from build123d import *

# Parameters (mm, degrees)
SKETCH1_W           = 100
SKETCH1_H           = 80
BOSS_EXTRUDE1_DEPTH = 30
SKETCH2_W           = 23.5
SKETCH2_H           = 28.5
SKETCH2_W_2         = 27
CUT_EXTRUDE1_DEPTH  = 25
SKETCH3_W           = 80
SKETCH3_H           = 60
CUT_EXTRUDE2_DEPTH  = 3
SKETCH5_W           = 89
SKETCH5_H           = 69
SKETCH5_W_2         = 80
SKETCH5_H_2         = 60
BOSS_EXTRUDE2_DEPTH = 7
FILLET1_R           = 3


with BuildPart() as part:
    # Sketch1 → Boss-Extrude1 (new body)
    with BuildSketch(Plane(origin=(0, 0, 0), x_dir=(1, 0, 0), z_dir=(0, 1, 0))):
        Rectangle(SKETCH1_W, SKETCH1_H)
    extrude(amount=BOSS_EXTRUDE1_DEPTH)

    # Sketch2 → Cut-Extrude1 (cut)
    with BuildSketch(Plane(origin=(0, 30, 0), x_dir=(1, 0, 0), z_dir=(0, 1, 0))):
        with Locations((-28.25, 15.75)):
            Rectangle(SKETCH2_W, SKETCH2_H)
        with Locations((0, 15.75)):
            Rectangle(SKETCH2_W_2, SKETCH2_H)
        with Locations((28.25, 15.75)):
            Rectangle(SKETCH2_W, SKETCH2_H)
        with Locations((28.25, -15.75)):
            Rectangle(SKETCH2_W, SKETCH2_H)
        with Locations((0, -15.75)):
            Rectangle(SKETCH2_W_2, SKETCH2_H)
        with Locations((-28.25, -15.75)):
            Rectangle(SKETCH2_W, SKETCH2_H)
    extrude(amount=-CUT_EXTRUDE1_DEPTH, mode=Mode.SUBTRACT)

    # Sketch3 → Cut-Extrude2 (cut)
    with BuildSketch(Plane(origin=(0, 30, 0), x_dir=(1, 0, 0), z_dir=(0, 1, 0))):
        Rectangle(SKETCH3_W, SKETCH3_H)
    extrude(amount=-CUT_EXTRUDE2_DEPTH, mode=Mode.SUBTRACT)

    # Sketch5 → Boss-Extrude2 (add)
    with BuildSketch(Plane(origin=(0, 30, 0), x_dir=(1, 0, 0), z_dir=(0, 1, 0))):
        Rectangle(SKETCH5_W, SKETCH5_H)
        Rectangle(SKETCH5_W_2, SKETCH5_H_2, mode=Mode.SUBTRACT)
    extrude(amount=BOSS_EXTRUDE2_DEPTH)

    # Fillet1
    fillet1_edges = [part.edges().sort_by_distance(p)[0] for p in [
        (-44.5, 33.5, -34.5),
        (-44.5, 33.5, 34.5),
        (44.5, 33.5, 34.5),
        (44.5, 33.5, -34.5),
    ]]
    fillet(fillet1_edges, radius=FILLET1_R)


solid = part.part
Verification items for the finished model (mm, model axes). A direction names the side the tool comes from. Coordinates: 2 decimals unless noted, no trailing zeros. Order: outer loops, then holes, each group sorted by start corner. A loop starts at its lowest first (then second) coordinate and runs counter-clockwise, first axis right, second up. Notation, with made-up numbers: M 60,39.5 L 84,39.5 A18 ccw 84,62.5 Z; hole C 73,5 d5. An arc over 180 degrees is marked long. One line per item, written item: value. Start each with the question number.
Item 1: Access from +Z, -Z, +X, -X, +Y, -Y to the whole of each face (thin tool, end or side, straight path). Record for faces 4 (the flat face through (-1, 15, 40)), 5 (the flat face through (44.5, 33, 0)), 6 (the flat face through (-44.5, 33, 0)), 7 (the cylindrical face through (-43.64, 33.55, -33.6)), 8 (the flat face through (-13.5, 16, 16)).
Item 2: Sectioned sample at B-B on y = 28.5. Record the cut outline in (x, z), then the cut area to 3 significant figures.
Item 3: Thickness scan on probe 1 along Z at (x, y) = (-17, 8); probe 2 along X at (y, z) = (13.5, -20.5); probe 3 along Z at (x, y) = (13, 28). Record the ranges inside material, lowest first.
Item 4: Mould release check, pull along X, two halves, no side actions. Record for faces 1 (the cylindrical face through (43.64, 33.55, -33.6)), 2 (the flat face through (-1, 33, 34.5)), 3 (the flat face through (0, 27, 0)): pulls with the +X half, pulls with the -X half, needs draft (parallel to the pull), parting line crosses it, or undercut.
Item 5: Sectioned sample at A-A on y = 18.5. Record the cut outline in (x, z), then the cut area to 3 significant figures.
Item 6: Depth check by flat-ended pin: P1, Ø4, axis at x = 15, z = -9.5, coming from the +Y side; P2, Ø12, axis at x = -24.5, z = 14.5, coming from the +Y side; P3, Ø3.5, axis at x = 15, y = 34.5, coming from the +Z side. Enter the tip coordinate at first touch or a pass-through.
Item 7: Sectioned sample at C-C on z = -4.5. Record the cut outline in (x, y), then the cut area to 4 significant figures.
Item 8: Sectioned sample at D-D on x = 4. Record the cut outline in (y, z).
Calculated:
1. face 4: +Z, +X, -X, +Y, -Y
1. face 5: +Z, -Z, +X, +Y
1. face 6: +Z, -Z, -X, +Y
1. face 7: -Z, -X, +Y
1. face 8: +Y
2. outline: M -50,-40 L 50,-40 L 50,40 L -50,40 Z; hole M -40,-30 L 40,-30 L 40,30 L -40,30 Z
2. area: 3,200 mm^2
3. probe 1: -40 to -30, -1.5 to 1.5, 30 to 40
3. probe 2: -50 to -40, -16.5 to -13.5, 13.5 to 16.5, 40 to 50
3. probe 3: -40 to -30, 30 to 40
4. face 1: pulls with the +X half
4. face 2: needs draft
4. face 3: undercut
5. outline: M -50,-40 L 50,-40 L 50,40 L -50,40 Z; hole M -40,-30 L -16.5,-30 L -16.5,-1.5 L -40,-1.5 Z; hole M -40,1.5 L -16.5,1.5 L -16.5,30 L -40,30 Z; hole M -13.5,-30 L 13.5,-30 L 13.5,-1.5 L -13.5,-1.5 Z; hole M -13.5,1.5 L 13.5,1.5 L 13.5,30 L -13.5,30 Z; hole M 16.5,-30 L 40,-30 L 40,-1.5 L 16.5,-1.5 Z; hole M 16.5,1.5 L 40,1.5 L 40,30 L 16.5,30 Z
5. area: 3,780 mm^2
6. P1: y = 27
6. P2: y = 5
6. P3: z = 34.5
7. outline: M -50,0 L 50,0 L 50,30 L 44.5,30 L 44.5,37 L 40,37 L 40,5 L 16.5,5 L 16.5,27 L 13.5,27 L 13.5,5 L -13.5,5 L -13.5,27 L -16.5,27 L -16.5,5 L -40,5 L -40,37 L -44.5,37 L -44.5,30 L -50,30 Z
7. area: 1,195 mm^2
8. outline: M 0,-40 L 30,-40 L 30,-34.5 L 37,-34.5 L 37,-30 L 5,-30 L 5,-1.5 L 27,-1.5 L 27,1.5 L 5,1.5 L 5,30 L 37,30 L 37,34.5 L 30,34.5 L 30,40 L 0,40 Z
